Check sheet for the drawn part. Datum: minimum x, y, z corner. Units: mm. Give positions to 0.01 mm unless a question says otherwise; leave off trailing zeros. Order: outer loops, then holes, each group sorted by start corner. A loop starts at its lowest first (then second) coordinate and runs counter-clockwise, first axis right, second up.
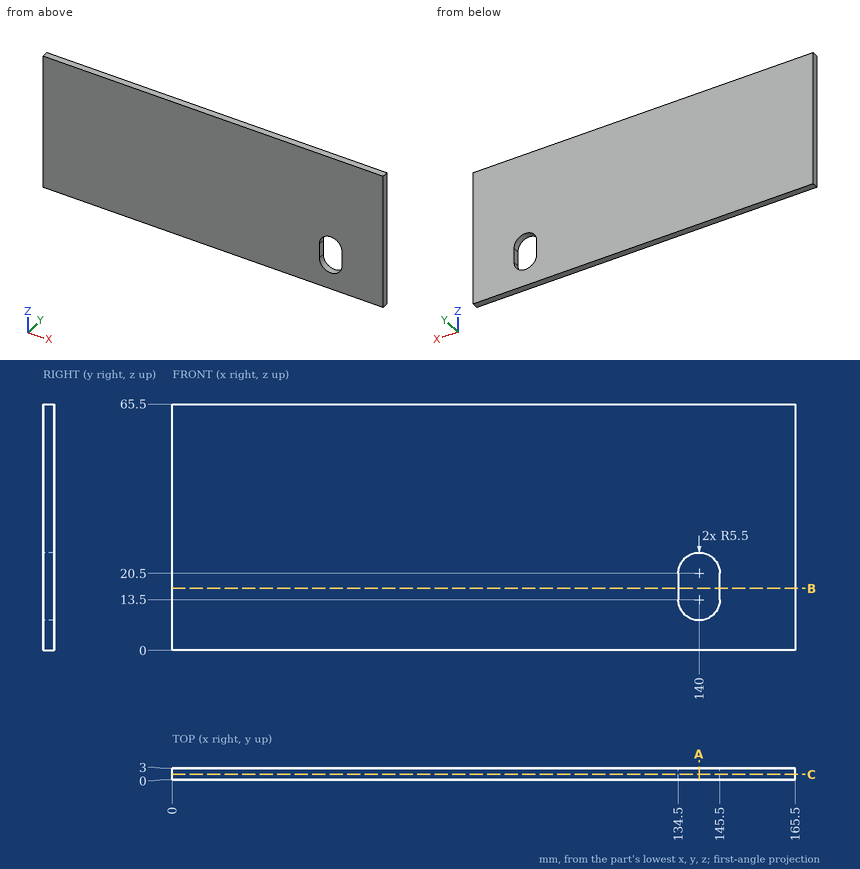
Q1. Sectioned sample at A-A, the plane x = 140. Record the cut outline in (y, z).
Q2. Sectioned sample at C-C, the plane y = 1.4. Record the cut outline in (x, z).
Q3. Sectioned sample at B-B, the plane z = 16.5. Record the cut outline in (x, y), plus the area to 4 significant figures.
Q4. Material ranges on line 1 (Z direction, x = 139.5, y = 0.75); line 2 (X direction, y = 0.4, z = 15); line 3 (X direction, y = 2.2, z = 22), recorded low to high.
Filled in:
1. outline: (0, 0) - (3, 0) - (3, 8) - (0, 8) - close; (0, 26) - (3, 26) - (3, 65.5) - (0, 65.5) - close
2. outline: (0, 0) - (165.5, 0) - (165.5, 65.5) - (0, 65.5) - close; hole (134.5, 13.5) arc R5.5 ccw to (145.5, 13.5) - (145.5, 20.5) arc R5.5 ccw to (134.5, 20.5) - close
3. outline: (0, 0) - (134.5, 0) - (134.5, 3) - (0, 3) - close; (145.5, 0) - (165.5, 0) - (165.5, 3) - (145.5, 3) - close
3. area: 463.5 mm2
4. line 1: z = 0 to 8.02, 25.98 to 65.5
4. line 2: x = 0 to 134.5, 145.5 to 165.5
4. line 3: x = 0 to 134.71, 145.29 to 165.5
